Can you work these out from the model? Positions are in its coordinate system, mm. Face numbers are marked on the shaded views. A direction names the side the tool comes from. Coordinates: 2 decimals unless noted, no trailing zeros. Order: outer loops, then holes, each group sorted by start corner. A loop starts at its lowest first (then second) coordinate and runs counter-clockwise, first axis right, second up.
```python
from build123d import *

# Parameters (mm, degrees)
EXTRUDE_1_DEPTH     = 3
EXTRUDE_2_DEPTH     = 77
SKETCH_3_W          = 96
SKETCH_3_H          = 2
EXTRUDE_3_DEPTH     = 30
CUT_EXTRUDE_1_DEPTH = 164.474768695
EXTRUDE_4_DEPTH     = 3
SKETCH_8_R          = 2
CUT_EXTRUDE_2_DEPTH = 3
SKETCH_9_R          = 1.15
CUT_EXTRUDE_3_DEPTH = 23
SKETCH_10_W         = 1
SKETCH_10_H         = 68
CUT_EXTRUDE_4_DEPTH = 1
SKETCH_11_W         = 100
SKETCH_11_H         = 1.130513839
SKETCH_11_H_2       = 1
CUT_EXTRUDE_5_DEPTH = 1


with BuildPart() as part:
    # 草图1 → 凸台-拉伸1 (new body)
    with BuildSketch(Plane(origin=(0, 0, 0), x_dir=(1, 0, 0), z_dir=(0, 1, 0))):
        with BuildLine():
            Line((0, 0), (0, -20))
            Line((0, -20), (60, -20))
            ThreePointArc((60, -20), (74, -34), (60, -48))
            Line((60, -48), (0, -48))
            Line((0, -48), (0, -68))
            Line((0, -68), (100, -68))
            Line((100, -68), (100, 0))
            Line((100, 0), (0, 0))
        make_face()
    extrude(amount=EXTRUDE_1_DEPTH)

    # 草图2 → 凸台-拉伸2 (add)
    with BuildSketch(Plane(origin=(0, 3, 0), x_dir=(1, 0, 0), z_dir=(0, 1, 0))):
        Polygon((2, -20), (0, -20), (0, 0), (100, 0), (100, -68), (0, -68), (0, -48), (2, -48), (2, -66), (98, -66), (98, -2), (2, -2), align=None)
    extrude(amount=EXTRUDE_2_DEPTH)

    # 草图3 → 凸台-拉伸3 (add)
    with BuildSketch(Plane(origin=(0, 80, 0), x_dir=(1, 0, 0), z_dir=(0, 1, 0))):
        with Locations((50, -1)):
            Rectangle(SKETCH_3_W, SKETCH_3_H)
        with Locations((50, -67)):
            Rectangle(SKETCH_3_W, SKETCH_3_H)
    extrude(amount=EXTRUDE_3_DEPTH)

    # 草图6 → 切除-拉伸1 (cut, through all)
    with BuildSketch(Plane.XY.offset(68)):
        Polygon((2, 110), (2, 80), (98, 110), align=None)
    extrude(amount=-CUT_EXTRUDE_1_DEPTH, mode=Mode.SUBTRACT)

    # 草图7 → 凸台-拉伸4 (add)
    with BuildSketch(Plane(origin=(0, 3, 0), x_dir=(1, 0, 0), z_dir=(0, 1, 0))):
        with BuildLine():
            Line((98, -2), (2, -2))
            Line((2, -2), (2, -20))
            Line((2, -20), (60, -20))
            ThreePointArc((60, -20), (74, -34), (60, -48))
            Line((60, -48), (2, -48))
            Line((2, -48), (2, -66))
            Line((2, -66), (98, -66))
            Line((98, -66), (98, -2))
        make_face()
    extrude(amount=EXTRUDE_4_DEPTH)

    # 草图8 → 切除-拉伸2 (cut)
    with BuildSketch(Plane(origin=(0, 6, 0), x_dir=(1, 0, 0), z_dir=(0, 1, 0))):
        with Locations(Location((15, -9, 0), (0, 0, 270))):
            Circle(SKETCH_8_R)
        with Locations(Location((50, -9, 0), (0, 0, 270))):
            Circle(SKETCH_8_R)
        with Locations(Location((85, -9, 0), (0, 0, 270))):
            Circle(SKETCH_8_R)
        with Locations(Location((15, -59, 0), (0, 0, 270))):
            Circle(SKETCH_8_R)
        with Locations(Location((50, -59, 0), (0, 0, 270))):
            Circle(SKETCH_8_R)
        with Locations(Location((85, -59, 0), (0, 0, 270))):
            Circle(SKETCH_8_R)
    extrude(amount=-CUT_EXTRUDE_2_DEPTH, mode=Mode.SUBTRACT)

    # 草图9 → 切除-拉伸3 (cut)
    with BuildSketch(Plane(origin=(0, 6, 0), x_dir=(1, 0, 0), z_dir=(0, 1, 0))):
        with Locations(Location((15, -9, 0), (0, 0, 270))):
            Circle(SKETCH_9_R)
        with Locations(Location((50, -9, 0), (0, 0, 270))):
            Circle(SKETCH_9_R)
        with Locations(Location((85, -9, 0), (0, 0, 270))):
            Circle(SKETCH_9_R)
        with Locations(Location((85, -59, 0), (0, 0, 270))):
            Circle(SKETCH_9_R)
        with Locations(Location((50, -59, 0), (0, 0, 270))):
            Circle(SKETCH_9_R)
        with Locations(Location((15, -59, 0), (0, 0, 270))):
            Circle(SKETCH_9_R)
    extrude(amount=-CUT_EXTRUDE_3_DEPTH, mode=Mode.SUBTRACT)

    # 草图10 → 切除-拉伸4 (cut)
    with BuildSketch(Plane.XZ):
        with Locations((24.5, 34)):
            Rectangle(SKETCH_10_W, SKETCH_10_H)
        with Locations((39.5, 34)):
            Rectangle(SKETCH_10_W, SKETCH_10_H)
        with Locations((60.5, 34)):
            Rectangle(SKETCH_10_W, SKETCH_10_H)
        with Locations((75.5, 34)):
            Rectangle(SKETCH_10_W, SKETCH_10_H)
        with Locations((95.5, 34)):
            Rectangle(SKETCH_10_W, SKETCH_10_H)
        with Locations((4.5, 34)):
            Rectangle(SKETCH_10_W, SKETCH_10_H)
    extrude(amount=-CUT_EXTRUDE_4_DEPTH, mode=Mode.SUBTRACT)

    # 草图11 → 切除-拉伸5 (cut)
    with BuildSketch(Plane.XZ):
        with Locations((50, 47.43474308)):
            Rectangle(SKETCH_11_W, SKETCH_11_H)
        with Locations((50, 20.5)):
            Rectangle(SKETCH_11_W, SKETCH_11_H_2)
    extrude(amount=-CUT_EXTRUDE_5_DEPTH, mode=Mode.SUBTRACT)


solid = part.part
```
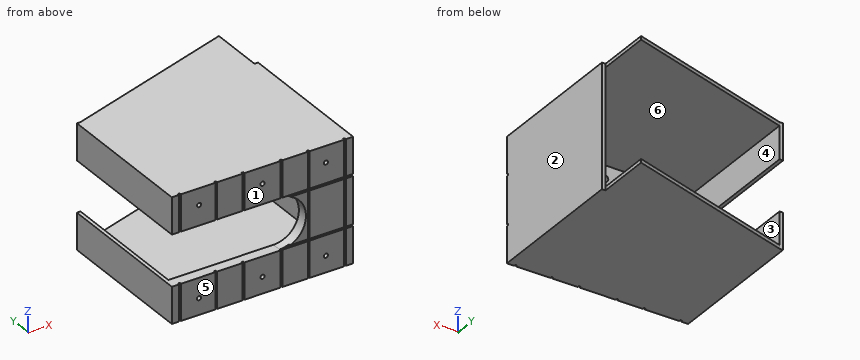
1. Imagine slicing it at C-C on z = 34. Please give me the cut outline in (x, y).
Completed:
outline: (74, 0) - (75, 0) - (75, 1) - (76, 1) - (76, 0) - (95, 0) - (95, 1) - (96, 1) - (96, 0) - (100, 0) - (100, 80) - (98, 80) - (98, 6) - (74, 6) - close
2. On a 3-axis mill with a long thin cutter (end or side, diameter ignored), from which of +Z, -Z, +X, -X, +Y, -Y can I reach the whole of each face in a straight line? I mean the marked faces 5 and 6. Say none if no direction works.
Completed:
face 5: +Z, -Z, +X, -X, -Y
face 6: +Y
3. Imagine slicing it at A-A on y = 69. Please give me the cut outline in (x, z).
Completed:
outline: (0, 0) - (100, 0) - (100, 68) - (0, 68) - (0, 48) - (2, 48) - (2, 66) - (98, 66) - (98, 2) - (2, 2) - (2, 20) - (0, 20) - close
4. Please list where these lines run through material, in increasing order: probe 1 along X at (y, z) = (1.6, 59); probe 2 along Z at (x, y) = (85, 1.9); probe 3 along X at (y, z) = (73.5, 65).
Completed:
probe 1: x = 0 to 13.85, 16.15 to 48.85, 51.15 to 83.85, 86.15 to 100
probe 2: z = 0 to 7.85, 10.15 to 57.85, 60.15 to 68
probe 3: x = 0 to 2, 98 to 100
5. Thinking about a two-plate mould opening in X: for the marked faces 1, 2, 3 and 4, which applies, pulls with the +X half, pulls with the -X half, needs draft (parallel to the pull), parting line crosses it, or undercut?
Completed:
face 1: needs draft
face 2: pulls with the +X half
face 3: undercut
face 4: undercut
6. I'm going to push flat-ended pins straight in: pin 1 (3 mm diameter, centred on x = 16, z = 59.5, fed in from +Y); pin 2 (0.5 mm diameter, centred on x = 4.5, z = 12.5, fed in from -Y); pin 3 (3.5 mm diameter, centred on x = 85, z = 59, fed in from +Y). Where does each tip first touch, or does it pass through?
Completed:
pin 1: stops at y = 6
pin 2: stops at y = 1
pin 3: stops at y = 3
